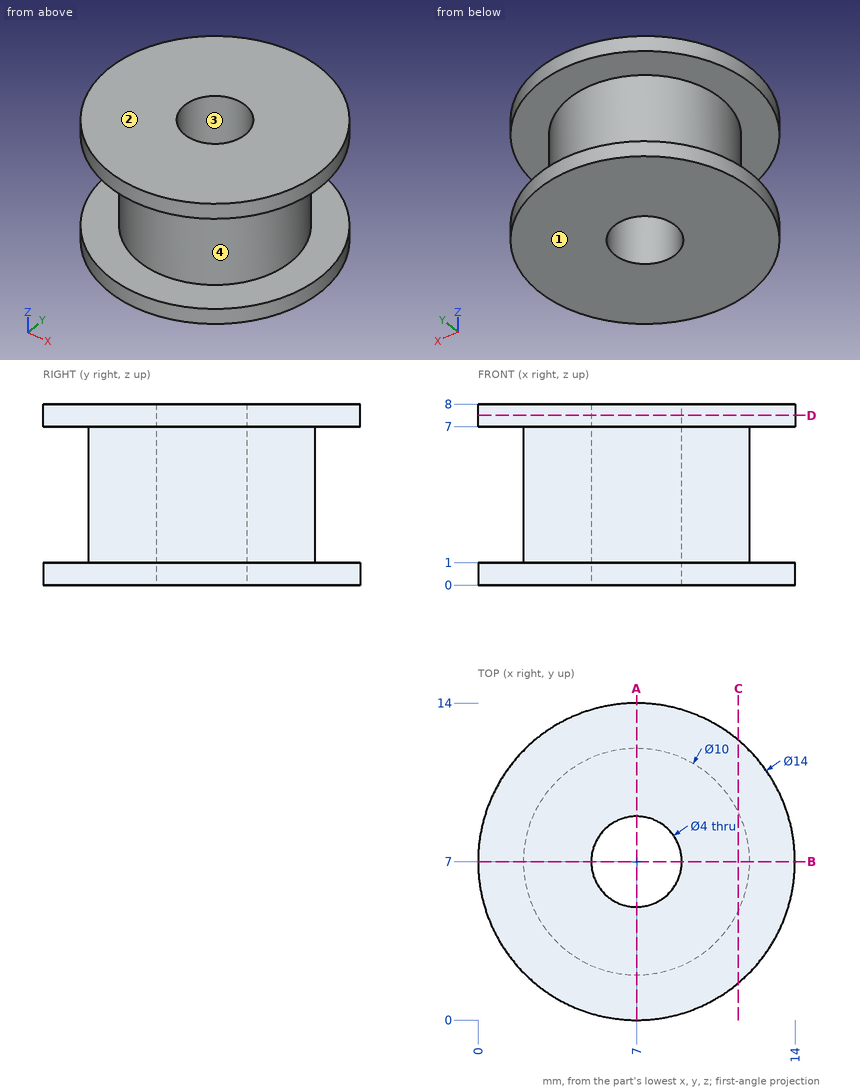
Part print with two shaded views. Sizes in mm from the minimum x, y, z corner. Round coordinates to 2 decimals unless told otherwise and drop trailing zeros. Order: outer loops, then holes, each group sorted by start corner. A loop starts at its lowest first (then second) coordinate and runs counter-clockwise, first axis right, second up. Notation, with made-up numbers: M 34,35 L 81,35 A12 cw 81,45 Z; hole C 35,-7.5 d2. An arc over 180 degrees is marked long. Put each result on its own line as item: value. Start each with the question number.
1. Drill centre lines: probe 1 along Y at (x, z) = (7, 3); probe 2 along Z at (x, y) = (10.5, 1); probe 3 along Y at (x, z) = (5.75, 6). Where is each one in solid material? Low to high. Write a range as [from, to].
2. Two-plate mould, pull along Z, no slides. Class the marked faces 1, 2, 3 and 4: +Z half, -Z half, draft (parallel to the pull), parting line (faces both ways), or undercut.
3. Slice it at D-D on z = 7.5. List the corners of the cut face in (x, y).
4. Drop flat-ended pins along their axis: pin 1 (2 mm diameter, centred on y = 4, z = 5, fed in from +X); pin 2 (3.5 mm diameter, centred on x = 7, y = 7, fed in from -Z). Give the stop position or say it passes through.
5. Slice it at A-A on x = 7. List the corners of the cut face in (y, z), then the cut area to 3 significant figures.
6. Slice it at C-C on x = 11.5. List the corners of the cut face in (y, z).
Findings:
1. probe 1: [2, 5], [9, 12]
1. probe 2: [0, 1], [7, 8]
1. probe 3: [2.16, 5.44], [8.56, 11.84]
2. face 1: -Z half
2. face 2: +Z half
2. face 3: draft
2. face 4: undercut
3. outline: C 7,7 d14; hole C 7,7 d4
4. pin 1: x = 11.58
4. pin 2: through
5. outline: M 0,0 L 5,0 L 5,8 L 0,8 L 0,7 L 2,7 L 2,1 L 0,1 Z; M 9,0 L 14,0 L 14,1 L 12,1 L 12,7 L 14,7 L 14,8 L 9,8 Z
5. area: 56.0 mm2
6. outline: M 1.64,0 L 12.36,0 L 12.36,1 L 9.18,1 L 9.18,7 L 12.36,7 L 12.36,8 L 1.64,8 L 1.64,7 L 4.82,7 L 4.82,1 L 1.64,1 Z
